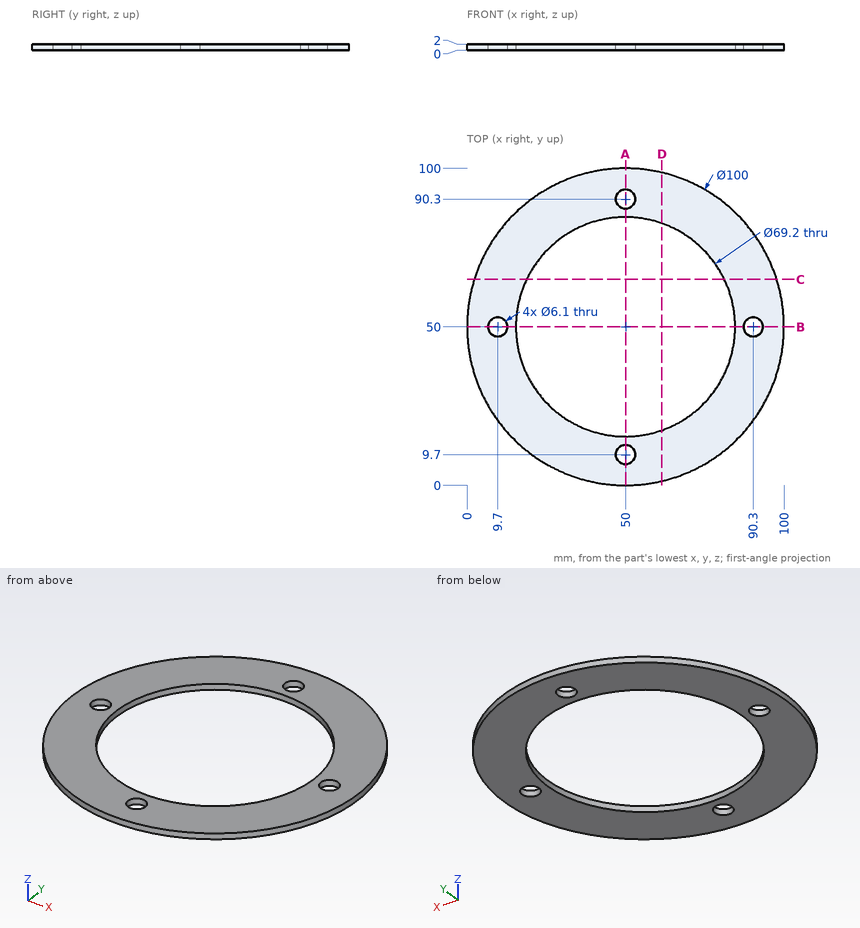
Design review of the part shown in the three views and the two pictorial views. Dimensions are in mm from the part's minimum x, y and z. Round coordinates to 2 decimals unless told otherwise and drop trailing zeros. Loops run counter-clockwise (first coordinate to the right, second up) from the corner with the lowest first, then second, coordinate; pieces in that order, holes last. Notation, with made-up numbers: (32, 82) - (52, 82) arc R25 ccw to (52, 109) - close; hole circle Ø9 at (50, -9). An arc over 180 degrees is marked (long way). Use one line per item in the form item = value.
1) We need section C-C on y = 65. Write out the cut boundary in (x, z).
Solutions:
outline = (2.3, 0) - (18.82, 0) - (18.82, 2) - (2.3, 2) - close; (81.18, 0) - (97.7, 0) - (97.7, 2) - (81.18, 2) - close
2) Clearance check with flat-ended pins moving along their axes: P1, Ø7, axis at x = 9.7, y = 50, coming from the -Z side; P2, Ø1, axis at x = 57.5, z = 1.5, coming from the -Y side. State where each tip first meets the part, or that it passes through.
Solutions:
P1 = 0
P2 = 0.49
3) We need section D-D on x = 61.5. Write out the cut boundary in (y, z).
Solutions:
outline = (1.34, 0) - (17.37, 0) - (17.37, 2) - (1.34, 2) - close; (82.63, 0) - (98.66, 0) - (98.66, 2) - (82.63, 2) - close
4) Wall thickness on probe 1 along X at (y, z) = (50, 0.5); probe 2 along Y at (x, z) = (52.5, 1.35): over which ranges is each line inside the solid? List them lowest first.
Solutions:
probe_1 = 0 to 6.65, 12.75 to 15.4, 84.6 to 87.25, 93.35 to 100
probe_2 = 0.06 to 7.95, 11.45 to 15.49, 84.51 to 88.55, 92.05 to 99.94
5) We need section A-A on x = 50. Write out the cut boundary in (y, z).
Solutions:
outline = (0, 0) - (6.65, 0) - (6.65, 2) - (0, 2) - close; (12.75, 0) - (15.4, 0) - (15.4, 2) - (12.75, 2) - close; (84.6, 0) - (87.25, 0) - (87.25, 2) - (84.6, 2) - close; (93.35, 0) - (100, 0) - (100, 2) - (93.35, 2) - close
